CAD build for the part. Positions are in the model's coordinates, mm. Round coordinates to 2 decimals unless told otherwise and drop trailing zeros. Write item = value, one per line.
from build123d import *

# Parameters (mm, degrees)
SKETCH3_R           = 19.898430298
BOSS_EXTRUDE1_DEPTH = 6.35
BOSS_EXTRUDE2_DEPTH = 6.35
CIRPATTERN1_COUNT   = 16
SKETCH5_R           = 12.7
CUT_EXTRUDE1_DEPTH  = 41.290772811


with BuildPart() as part:
    # Sketch3 → Boss-Extrude1 (new body)
    with BuildSketch(Plane(origin=(0, 0, 0), x_dir=(1, 0, 0), z_dir=(0, 1, 0))):
        with Locations(Location((0, 0, 0), (0, 0, 270))):
            Circle(SKETCH3_R)
    extrude(amount=BOSS_EXTRUDE1_DEPTH)

    # Sketch4 → Boss-Extrude2 (add)
    with BuildSketch(Plane(origin=(0, 0, 0), x_dir=(1, 0, 0), z_dir=(0, 1, 0))):
        with BuildLine():
            Line((1.988478018, 20.052825306), (1.988478018, 19.798825306))
            ThreePointArc((1.988478018, 19.798825306), (-1.950387235, 19.802613917), (-5.812829174, 19.030463612))
            Line((-5.812829174, 19.030463612), (-5.862382116, 19.279583074))
            add(Edge.make_bspline(
                [(-2.898476267, 28.108453205), (-3.6130336, 27.120887472), (-5.51050926, 24.413306859), (-6.393741318, 21.275894599), (-5.862382116, 19.279583074)],
                knots=[0.009892854, 0.009892854, 0.009892854, 0.009892854, 0.401482073, 1, 1, 1, 1], degree=3))
            ThreePointArc((-2.898476267, 28.108453205), (-2.769719343, 28.121432414), (-2.640904329, 28.133821827))
            add(Edge.make_bspline(
                [(-2.640904329, 28.133821827), (-1.747412498, 27.304635113), (-0.175879044, 25.791834729), (1.64701783, 23.095158006), (1.988478018, 21.20759249), (1.988478018, 20.052825306)],
                knots=[0.009892854, 0.009892854, 0.009892854, 0.009892854, 0.401482073, 0.665435678, 1, 1, 1, 1], degree=3))
        make_face()
    boss_extrude2 = extrude(amount=BOSS_EXTRUDE2_DEPTH)

    # CirPattern1: Boss-Extrude2 ×16 about axis
    cirpattern1_axis = Axis((0, 6.35, 0), (0, -1, 0))
    for i in range(1, CIRPATTERN1_COUNT):
        add(boss_extrude2.rotate(cirpattern1_axis, i * 360 / CIRPATTERN1_COUNT))

    # Sketch5 → Cut-Extrude1 (cut, through all)
    with BuildSketch(Plane(origin=(0, 6.35, 0), x_dir=(1, 0, 0), z_dir=(0, 1, 0))):
        with Locations(Location((0, 0, 0), (0, 0, 270))):
            Circle(SKETCH5_R)
    extrude(amount=-CUT_EXTRUDE1_DEPTH, mode=Mode.SUBTRACT)


solid = part.part
(1) Probe line 1 along Z through (x, y) = (24, 5.5); line 2 along X through (y, z) = (5.5, -7.5); line 3 along X through (y, z) = (3.5, 19). List the from-to ranges inside material, lowest first.
Solved:
line_1 = -13.63 to -10.79, -5.39 to 0.98, 3.98 to 9.55
line_2 = -26.72 to -10.25, 10.25 to 21.87
line_3 = -18.04 to -10.41, -9.93 to 14.11
(2) Drop flat-ended pins along their axis: pin 1 (2 mm diameter, centred on y = 3, z = -2.5, fed in from -X); pin 2 (2 mm diameter, centred on y = 4, z = 20, fed in from +X); pin 3 (3 mm diameter, centred on x = 11, y = 3, fed in from +Z); pin 4 (6 mm diameter, centred on x = 8.5, z = -5, fed in from -Y). Give the stop position or say it passes through.
Solved:
pin_1 = -23.46
pin_2 = 14.16
pin_3 = 24.72
pin_4 = 0
(3) Band-saw the part on A-A on z = 23. Count the separate pieces of the cut face and the enclosed holes in it, plus the area to 3 significant figures.
Solved:
separate_pieces = 3
enclosed_holes = 0
area = 120 mm²
(4) Pull direction Z, two halves, no side cores. Call faces 1 (the cylindrical face through (-7.7, 3.2, -10.1)), 2 (the flat face through (8.8, 0, -9.4)): released by +Z, released by -Z, zero draft, split by the parting line, or undercut.
Solved:
face_1 = undercut
face_2 = zero draft
